```python
from build123d import *

# Parameters (mm, degrees)
SKETCH1_W               = 50.8
SKETCH1_H               = 54.61
BOSS_EXTRUDE1_DEPTH     = 5.08
BOSS_EXTRUDE2_DEPTH     = 54.61
CUT_EXTRUDE1_DEPTH      = 75.911162886
CUT_EXTRUDE1_DEPTH_BACK = 5.08
SKETCH4_W               = 50.8
SKETCH4_H               = 15.24
BOSS_EXTRUDE3_DEPTH     = 5.08
CUT_EXTRUDE2_REACH      = 74.025
SKETCH5_W               = 6.985
SKETCH5_H               = 12.7
CUT_EXTRUDE3_START      = -15.24
SKETCH6_W               = 40
SKETCH6_H               = 15.24
CUT_EXTRUDE3_DEPTH      = 15.24
SKETCH8_W               = 15.24
SKETCH8_H               = 5.08
BOSS_EXTRUDE4_DEPTH     = 5.08
SKETCH9_R               = 2.5
CUT_EXTRUDE4_DEPTH      = 5.08


with BuildPart() as part:
    # Sketch1 → Boss-Extrude1 (new body)
    with BuildSketch(Plane.XY):
        with Locations((25.4, 27.305)):
            Rectangle(SKETCH1_W, SKETCH1_H)
    extrude(amount=BOSS_EXTRUDE1_DEPTH)

    # Sketch2 → Boss-Extrude2 (add)
    with BuildSketch(Plane.XZ):
        Polygon((10.668, 5.08), (6.380565044, 5.08), (6.380565044, 12.065), (16.256, 12.065), align=None)
        Polygon((34.544, 12.065), (40.132, 5.08), (44.419434956, 5.08), (44.419434956, 12.065), align=None)
    extrude(amount=-BOSS_EXTRUDE2_DEPTH)

    # Sketch3 → Cut-Extrude1 (cut, two sides: drawn at the far end of the back side and taken through both)
    with BuildSketch(Plane.XY.offset(5.08).offset(-CUT_EXTRUDE1_DEPTH_BACK)):
        with BuildLine():
            Line((22.32, 48.8), (22.32, 14.7))
            ThreePointArc((22.32, 14.7), (20.32, 12.7), (18.32, 14.7))
            Line((18.32, 14.7), (18.32, 48.8))
            ThreePointArc((18.32, 48.8), (20.32, 50.8), (22.32, 48.8))
        make_face()
        with BuildLine():
            Line((28.48, 48.8), (28.48, 14.7))
            ThreePointArc((28.48, 14.7), (30.48, 12.7), (32.48, 14.7))
            Line((32.48, 14.7), (32.48, 48.8))
            ThreePointArc((32.48, 48.8), (30.48, 50.8), (28.48, 48.8))
        make_face()
    extrude(amount=CUT_EXTRUDE1_DEPTH + CUT_EXTRUDE1_DEPTH_BACK, mode=Mode.SUBTRACT)

    # Sketch4 → Boss-Extrude3 (add)
    with BuildSketch(Plane.XZ):
        with Locations((25.4, 7.62)):
            Rectangle(SKETCH4_W, SKETCH4_H)
    extrude(amount=BOSS_EXTRUDE3_DEPTH)

    # Cut-Extrude2: up to this face of the body (flat: up to its plane)
    cut_extrude2_end = Plane(part.part.faces().sort_by_distance((44.419434956, 27.305, 8.5725))[0])
    # Sketch5 → Cut-Extrude2 (cut, up to the picked face)
    with BuildSketch(Plane.ZY.offset(-6.380565044), mode=Mode.PRIVATE) as cut_extrude2_sk1:
        with Locations((8.5725, 6.35)):
            Rectangle(SKETCH5_W, SKETCH5_H)
    cut_extrude2_tool1 = split(extrude(cut_extrude2_sk1.sketch, amount=-CUT_EXTRUDE2_REACH, mode=Mode.PRIVATE), bisect_by=cut_extrude2_end, keep=Keep.BOTH, mode=Mode.PRIVATE)
    add(cut_extrude2_tool1.solids().sort_by(Axis((6.380565, 6.35, 8.5725), (1, 0, 0)))[0], mode=Mode.SUBTRACT)

    # Sketch6 → Cut-Extrude3 (cut)
    with BuildSketch(Plane.XY.offset(15.24).offset(CUT_EXTRUDE3_START)):
        with Locations((25.4, 2.54)):
            Rectangle(SKETCH6_W, SKETCH6_H)
    extrude(amount=CUT_EXTRUDE3_DEPTH, mode=Mode.SUBTRACT)

    # Sketch8 → Boss-Extrude4 (add)
    with BuildSketch(Plane.ZY):
        with Locations((7.62, -2.54)):
            Rectangle(SKETCH8_W, SKETCH8_H)
    boss_extrude4 = extrude(amount=BOSS_EXTRUDE4_DEPTH)

    # Mirror1: Boss-Extrude4 across plane
    add(boss_extrude4.mirror(Plane.ZY.offset(-25.4)))

    # Sketch9 → Cut-Extrude4 (cut)
    with BuildSketch(Plane(origin=(0, 0, 0), x_dir=(1, 0, 0), z_dir=(0, 1, 0))):
        with Locations(Location((0.16, -10.16, 0), (0, 0, 270))):
            Circle(SKETCH9_R)
        with Locations(Location((50.64, -10.16, 0), (0, 0, 90))):
            Circle(SKETCH9_R)
    extrude(amount=-CUT_EXTRUDE4_DEPTH, mode=Mode.SUBTRACT)


solid = part.part
```
Check sheet for the modelled part. Datum: model origin and axes. Units: mm. A direction names the side the tool comes from. Round coordinates to 2 decimals unless told otherwise and drop trailing zeros. Order: outer loops, then holes, each group sorted by start corner. A loop starts at its lowest first (then second) coordinate and runs counter-clockwise, first axis right, second up.
1) Section check D-D (z = 3). Record the boundary of the cut face in (x, y), and give its area (3 significant figures).
2) Tool access check on faces 1 (the flat face through (25, 10.16, 3)), 2 (the cylindrical face through (20.3, 50.8, 2.5)), 3 (the flat face through (37.3, 33.36, 8.62)). Record the directions out of +Z, -Z, +X, -X, +Y, -Y that give a thin tool (end or side, any length) a straight path to the whole face; none if there is none.
3) Mould release check, pull along X, two halves, no side actions. Record for faces 4 (the flat face through (41, 12.7, 9)), 5 (the cylindrical face through (20.4, 12.7, 2.5)), 6 (the flat face through (0, 28, 3)): +X half, -X half, draft (parallel to the pull), parting line (faces both ways), or undercut.
4) Section check A-A (y = 1.5). Record the boundary of the cut face in (x, z).
5) Section check C-C (y = 22.5). Record the boundary of the cut face in (x, z) (3 decimals), and give its area (3 significant figures).
6) Section check B-B (z = 13.5). Record the boundary of the cut face in (x, y), and give its area (3 significant figures).
7) Scan lines: line 1 (X direction, y = -1.7, z = 10.16); line 2 (X direction, y = 15, z = 3.5); line 3 (X direction, y = -1, z = 7.25). Record each from-to range of solid material in increasing order.
8) Go/stop test with flat-tipped pins: pin 1 Ø2 at (y, z) = (18.5, 7) entering from -X; pin 2 Ø1.5 at (y, z) = (40.5, 3.5) entering from +X; pin 3 Ø4 at (x, z) = (4, 10) entering from +Y. Record where each tip stops, or that it passes through.
Result:
1. outline: (-5.08, -5.08) - (5.4, -5.08) - (5.4, 10.16) - (45.4, 10.16) - (45.4, -5.08) - (55.88, -5.08) - (55.88, 0) - (50.8, 0) - (50.8, 54.61) - (0, 54.61) - (0, 0) - (-5.08, 0) - close; hole (18.32, 14.7) arc R2 ccw to (22.32, 14.7) - (22.32, 48.8) arc R2 ccw to (18.32, 48.8) - close; hole (28.48, 14.7) arc R2 ccw to (32.48, 14.7) - (32.48, 48.8) arc R2 ccw to (28.48, 48.8) - close
1. area: 2,180 mm2
2. face 1: +Z, -Z, -Y
2. face 2: +Z, -Z
2. face 3: +Y, -Y
3. face 4: draft
3. face 5: undercut
3. face 6: -X half
4. outline: (0, 0) - (5.4, 0) - (5.4, 5.08) - (0, 5.08) - close; (45.4, 0) - (50.8, 0) - (50.8, 5.08) - (45.4, 5.08) - close
5. outline: (0, 0) - (18.32, 0) - (18.32, 5.08) - (10.668, 5.08) - (16.256, 12.065) - (6.381, 12.065) - (6.381, 5.08) - (0, 5.08) - close; (22.32, 0) - (28.48, 0) - (28.48, 5.08) - (22.32, 5.08) - close; (32.48, 0) - (50.8, 0) - (50.8, 5.08) - (44.419, 5.08) - (44.419, 12.065) - (34.544, 12.065) - (40.132, 5.08) - (32.48, 5.08) - close
5. area: 316 mm2
6. outline: (-5.08, -5.08) - (5.4, -5.08) - (5.4, 0) - (-5.08, 0) - close; (45.4, -5.08) - (55.88, -5.08) - (55.88, 0) - (45.4, 0) - close
6. area: 106 mm2
7. line 1: x = -5.08 to -2.34, 2.66 to 5.4, 45.4 to 48.14, 53.14 to 55.88
7. line 2: x = 0 to 18.32, 22.32 to 28.48, 32.48 to 50.8
7. line 3: x = -5.08 to 5.4, 45.4 to 55.88
8. pin 1: stops at x = 6.38
8. pin 2: stops at x = 50.8
8. pin 3: stops at y = 0
